Design review of the part built by this model. Coordinates are the model's own, in mm. A direction names the side the tool comes from. Coordinates: 2 decimals unless noted, no trailing zeros. Loops run counter-clockwise (first coordinate to the right, second up) from the corner with the lowest first, then second, coordinate; pieces in that order, holes last. Notation, with made-up numbers: (-28, 64) - (7, 64) arc R17 cw to (7, 80) - close; hole circle Ø1 at (68, -37). An arc over 180 degrees is marked (long way). Answer in a Markdown table with one row per item. Add a question column.
(1) The part is to be moulded in two halves that separate along Y. For faces 1 (the face through (9.699, -9.715, -1.232)), 2 (the face through (6.758, 3.996, 4.54)), 3 (the face through (-8, -7.2, -0.5)), 4 (the face through (0, 10, -1)), say which applies: released by +Y, released by -Y, zero draft, split by the parting line, or undercut.
(2) We need section A-A, the plane z = -0.5. Write out the cut boundary in (x, y).
(3) To check wall thickness, follow L1, parallel to X at y = 2, z = -0.5; L2, parallel to Z at x = -5, y = 4. State the ranges of each line that lie inside material, in increasing order. Write a range as [from, to].
(4) We need section B-B, the plane x = 7.15. Write out the cut boundary in (y, z).
(5) For faces 5 (the face through (0.1, 8, -0.5)), 6 (the face through (0, 0, -2.5)), list the 3-axis set-ups (+Z, -Z, +X, -X, +Y, -Y) from which the entire face can be reached by the end or side of a thin tool; tool diameter is ignored.
(6) We need section C-C, the plane y = 4.75. Write out the cut boundary in (x, z).
(7) We need section D-D, the plane z = 1.5. Write out the cut boundary in (x, y).
(8) Clearance check with flat-ended pins moving along their axes: pin 1 (10 mm diameter, centred on x = 1, y = 4.5, fed in from +Z); pin 2 (2 mm diameter, centred on y = -4.5, z = 2, fed in from +X); pin 3 (5 mm diameter, centred on x = 1.5, y = 1.5, fed in from +Z). State where each tip first meets the part, or that it passes through.
Autodesk Inventor part; units mm, degrees
ref_plane "Cap_to_Frame_XY" through (0, 0, 0) normal (0, 0, -1) x (1, 0, 0)
ref_plane "Cap_to_Frame_YZ" through (0, 0, 0) normal (1, 0, 0) x (0, -1, 0)
ref_plane "Cap_to_Frame_ZX" through (0, 0, 0) normal (0, -1, 0) x (0, 0, -1)
sketch "Sketch_1" plane through (0, 0, 0) normal (0, 0, 1) x (1, 0, 0)
  arc A0 (-10, -9) -> (-9, -10) centre (-9, -9) ccw
  line L0 (-9, -10) -> (9, -10)
  arc A1 (9, -10) -> (10, -9) centre (9, -9) ccw
  line L1 (10, -9) -> (10, 9)
  arc A2 (10, 9) -> (9, 10) centre (9, 9) ccw
  line L2 (9, 10) -> (-9, 10)
  arc A3 (-9, 10) -> (-10, 9) centre (-9, 9) ccw
  line L3 (-10, 9) -> (-10, -9)
extrude "Extrusion1" add sketch "Sketch_1" against normal blind 2.5
sketch "Sketch_2" plane through (0, 0, 0) normal (0, 0, 1) x (1, 0, 0)
  arc A0 (-8, 6.3367) -> (-8, 3.1633) centre (-7.15, 4.75) ccw
  line L0 (-8, 3.1633) -> (-8, -3.1633)
  arc A1 (-8, -3.1633) -> (-8, -6.3367) centre (-7.15, -4.75) ccw
  line L1 (-8, -6.3367) -> (-8, -8)
  line L2 (-8, -8) -> (8, -8)
  line L3 (8, -8) -> (8, -6.3367)
  arc A2 (8, -6.3367) -> (8, -3.1633) centre (7.15, -4.75) ccw
  line L4 (8, -3.1633) -> (8, 3.1633)
  arc A3 (8, 3.1633) -> (8, 6.3367) centre (7.15, 4.75) ccw
  line L5 (8, 6.3367) -> (8, 8)
  line L6 (8, 8) -> (-8, 8)
  line L7 (-8, 8) -> (-8, 6.3367)
extrude "Extrusion2" cut sketch "Sketch_2" against normal blind 1
sketch "Sketch_3" plane through (0, 4.75, 0) normal (0, 1, 0) x (1, 0, 0)
  line L0 (-7.15, 1) -> (-7.15, -5.3)
  line L1 (-7.15, -5.3) -> (-8, -5.3)
  line L2 (-8, -5.3) -> (-8, -3.8)
  line L3 (-8, -3.8) -> (-8.15, -3.3)
  line L4 (-8.15, -3.3) -> (-8.15, 1)
  line L5 (-8.15, 1) -> (-7.15, 1)
  line L6 (-7.15, 1) -> (-7.15, -5.3)
revolve "Revolution1" add sketch "Sketch_3" angle 360 about axis through (-7.15, 4.75, -1) along (0, 0, -1)
pattern_linear "Rectangular Pattern1" count 2 spacing 14.3 along (1, 0, 0) count 2 spacing 9.5 along (0, -1, 0) of "Revolution1"
ref_plane "Cap_to_Frame_XY" through (0, 0, 0) normal (0, 0, -1) x (1, 0, 0)
ref_plane "Cap_to_Frame_YZ" through (0, 0, 0) normal (1, 0, 0) x (0, -1, 0)
ref_plane "Cap_to_Frame_ZX" through (0, 0, 0) normal (0, -1, 0) x (0, 0, -1)
properties part number "HFC5-2020-B"
Responses:
| question | item | result |
|---|---|---|
| 1 | face 1 | released by -Y |
| 1 | face 2 | undercut |
| 1 | face 3 | undercut |
| 1 | face 4 | released by +Y |
| 2 | outline | (-10, -9) arc R1 ccw to (-9, -10) - (9, -10) arc R1 ccw to (10, -9) - (10, 9) arc R1 ccw to (9, 10) - (-9, 10) arc R1 ccw to (-10, 9) - close; circle Ø2 at (-7.15, -4.75); circle Ø2 at (-7.15, 4.75); circle Ø2 at (7.15, -4.75); circle Ø2 at (7.15, 4.75); hole (-8, -8) - (8, -8) - (8, -6.34) arc R1.8 ccw to (8, -3.16) - (8, 3.16) arc R1.8 ccw to (8, 6.34) - (8, 8) - (-8, 8) - (-8, 6.34) arc R1.8 ccw to (-8, 3.16) - (-8, -3.16) arc R1.8 ccw to (-8, -6.34) - close |
| 3 | L1 | x = [-10, -8], [8, 10] |
| 3 | L2 | z = [-2.5, -1] |
| 4 | outline | (-10, -2.5) - (10, -2.5) - (10, 0) - (8, 0) - (8, -1) - (5.75, -1) - (5.75, 3.3) - (5.6, 3.8) - (5.6, 5.3) - (3.9, 5.3) - (3.9, 3.8) - (3.75, 3.3) - (3.75, -1) - (-3.75, -1) - (-3.75, 3.3) - (-3.9, 3.8) - (-3.9, 5.3) - (-5.6, 5.3) - (-5.6, 3.8) - (-5.75, 3.3) - (-5.75, -1) - (-8, -1) - (-8, 0) - (-10, 0) - close |
| 5 | face 5 | +Z |
| 5 | face 6 | -Z, +X, -X, +Y, -Y |
| 6 | outline | (-10, -2.5) - (10, -2.5) - (10, 0) - (8.95, 0) - (8.95, -1) - (8.15, -1) - (8.15, 3.3) - (8, 3.8) - (8, 5.3) - (6.3, 5.3) - (6.3, 3.8) - (6.15, 3.3) - (6.15, -1) - (-6.15, -1) - (-6.15, 3.3) - (-6.3, 3.8) - (-6.3, 5.3) - (-8, 5.3) - (-8, 3.8) - (-8.15, 3.3) - (-8.15, -1) - (-8.95, -1) - (-8.95, 0) - (-10, 0) - close |
| 7 | outline | circle Ø2 at (-7.15, -4.75); circle Ø2 at (-7.15, 4.75); circle Ø2 at (7.15, -4.75); circle Ø2 at (7.15, 4.75) |
| 8 | pin 1 | stops at z = 0 |
| 8 | pin 2 | stops at x = 8.15 |
| 8 | pin 3 | stops at z = -1 |
